```python
from build123d import *

# Parameters (mm, degrees)
SKETCH3_W                                        = 152.4
SKETCH3_H                                        = 15.875
BOSS_EXTRUDE1_DEPTH                              = 76.2
SKETCH4_R                                        = 22.621875
CUT_EXTRUDE1_DEPTH                               = 9.525
SKETCH5_R                                        = 18.0975
CUT_EXTRUDE2_DEPTH                               = 109.183203987
CBORE_FOR_1_4_SOCKET_HEAD_CAP_SCREW1_D           = 6.7564
CBORE_FOR_1_4_SOCKET_HEAD_CAP_SCREW1_CBORE_D     = 11.1125
CBORE_FOR_1_4_SOCKET_HEAD_CAP_SCREW1_CBORE_DEPTH = 6.35


with BuildPart() as part:
    # Sketch3 → Boss-Extrude1 (new, symmetric)
    with BuildSketch(Plane.XY):
        Rectangle(SKETCH3_W, SKETCH3_H)
    extrude(amount=BOSS_EXTRUDE1_DEPTH, both=True)

    # Sketch4 → Cut-Extrude1 (cut)
    with BuildSketch(Plane(origin=(0, 7.9375, 0), x_dir=(1, 0, 0), z_dir=(0, 1, 0))):
        with Locations(Location((0, 0, 0), (0, 0, 270))):
            Circle(SKETCH4_R)
    extrude(amount=-CUT_EXTRUDE1_DEPTH, mode=Mode.SUBTRACT)

    # Sketch5 → Cut-Extrude2 (cut, through all)
    with BuildSketch(Plane(origin=(0, -1.5875, 0), x_dir=(1, 0, 0), z_dir=(0, 1, 0))):
        with Locations(Location((0, 0, 0), (0, 0, 270))):
            Circle(SKETCH5_R)
    extrude(amount=-CUT_EXTRUDE2_DEPTH, mode=Mode.SUBTRACT)

    # CBORE for 1/4 Socket Head Cap Screw1 (through all)
    with Locations(Plane(origin=(-63.5, 7.9375, -33.866666667), x_dir=(0, 0, 1), z_dir=(0, 1, 0))):
        with Locations((0, 0), (-29.633333333, 38.1), (-29.633333333, 88.9), (0, 127), (67.733333334, 127), (97.366666667, 63.5), (67.733333334, 0)):
            CounterBoreHole(CBORE_FOR_1_4_SOCKET_HEAD_CAP_SCREW1_D / 2, CBORE_FOR_1_4_SOCKET_HEAD_CAP_SCREW1_CBORE_D / 2, CBORE_FOR_1_4_SOCKET_HEAD_CAP_SCREW1_CBORE_DEPTH)


solid = part.part
```
Check sheet for the modelled part. Datum: model origin and axes. Units: mm. A direction names the side the tool comes from. Round coordinates to 2 decimals unless told otherwise and drop trailing zeros. Write each loop counter-clockwise with the first axis right and the second up, starting at its lowest first coordinate (ties: lowest second). Pieces come first, ordered by that corner, then holes. Notation, with made-up numbers: (-17.75, -32.5) -> (8.25, -32.5) arc R18 cw to (8.25, -5.5) -> close; hole circle Ø2 at (89, -37.75). An arc over 180 degrees is marked (long way). Put each result on its own line as item: value.
(1) Sectioned sample at D-D (z = -63.5). Enter the section's corners in (x, y).
Values found:
outline: (-76.2, -7.94) -> (-28.78, -7.94) -> (-28.78, 1.59) -> (-30.96, 1.59) -> (-30.96, 7.94) -> (-76.2, 7.94) -> close; (-22.02, -7.94) -> (22.02, -7.94) -> (22.02, 1.59) -> (19.84, 1.59) -> (19.84, 7.94) -> (-19.84, 7.94) -> (-19.84, 1.59) -> (-22.02, 1.59) -> close; (28.78, -7.94) -> (76.2, -7.94) -> (76.2, 7.94) -> (30.96, 7.94) -> (30.96, 1.59) -> (28.78, 1.59) -> close
(2) Sectioned sample at B-B (x = -25.4). Enter the section's corners in (y, z), plus the area to 3 significant figures.
Values found:
outline: (-7.94, -76.2) -> (7.94, -76.2) -> (7.94, -69.06) -> (1.59, -69.06) -> (1.59, -66.88) -> (-7.94, -66.88) -> close; (-7.94, -60.12) -> (1.59, -60.12) -> (1.59, -57.94) -> (7.94, -57.94) -> (7.94, 76.2) -> (-7.94, 76.2) -> close
area: 2,280 mm^2
(3) Tool access check on faces 3 (the face through (15.2, -1.588, -10.2)), 4 (the face through (-66.798, -3.242, -33.134)). Record the directions out of +Z, -Z, +X, -X, +Y, -Y that give a thin tool (end or side, any length) a straight path to the whole face; none if there is none.
Values found:
face 3: +Y
face 4: +Y, -Y
(4) Mould release check, pull along X, two halves, no side actions. Record for faces 1 (the face through (-1, 0, -76.2)), 2 (the face through (-28, 1.588, -61)): released by +X, released by -X, zero draft, split by the parting line, or undercut.
Values found:
face 1: zero draft
face 2: undercut
(5) Sectioned sample at A-A (z = 63.5). Enter the section's corners in (x, y).
Values found:
outline: (-76.2, -7.94) -> (-3.38, -7.94) -> (-3.38, 1.59) -> (-5.56, 1.59) -> (-5.56, 7.94) -> (-76.2, 7.94) -> close; (3.38, -7.94) -> (76.2, -7.94) -> (76.2, 7.94) -> (5.56, 7.94) -> (5.56, 1.59) -> (3.38, 1.59) -> close
(6) Sectioned sample at C-C (y = 5.5). Count the separate pieces of the cut face and the enclosed holes in it, plus the area to 3 significant figures.
Values found:
separate pieces: 1
enclosed holes: 8
area: 20,900 mm^2
(7) Material ranges on line 1 (X direction, y = -4.25, z = -63.5); line 2 (Z direction, x = -64, y = 7); line 3 (Z direction, x = -62, y = 7), recorded low to high.
Values found:
line 1: x = -76.2 to -28.78, -22.02 to 22.02, 28.78 to 76.2
line 2: z = -76.2 to -39.4, -28.33 to 28.33, 39.4 to 76.2
line 3: z = -76.2 to -39.22, -28.52 to 28.52, 39.22 to 76.2
(8) Go/stop test with flat-tipped pins: pin 1 Ø5.5 at (x, z) = (64, 34) entering from +Y; pin 2 Ø11 at (x, z) = (63.5, 33.87) entering from +Y. Record where each tip stops, or that it passes through.
Values found:
pin 1: passes through
pin 2: stops at y = 1.59
